For this review, take the finished solid that the model builds, in its own axes (mm). Face numbers are marked on the shaded views. A direction names the side the tool comes from. Round coordinates to 2 decimals unless told otherwise and drop trailing zeros. Write each loop counter-clockwise with the first axis right and the second up, starting at its lowest first coordinate (ties: lowest second). Pieces come first, ordered by that corner, then holes. Notation, with made-up numbers: (-28, 74.25) - (9, 74.25) arc R4 ccw to (9, 79.25) - close; hole circle Ø5 at (26, 79.5). An arc over 180 degrees is marked (long way). Answer in a Markdown table with one row per item. Add a question column.
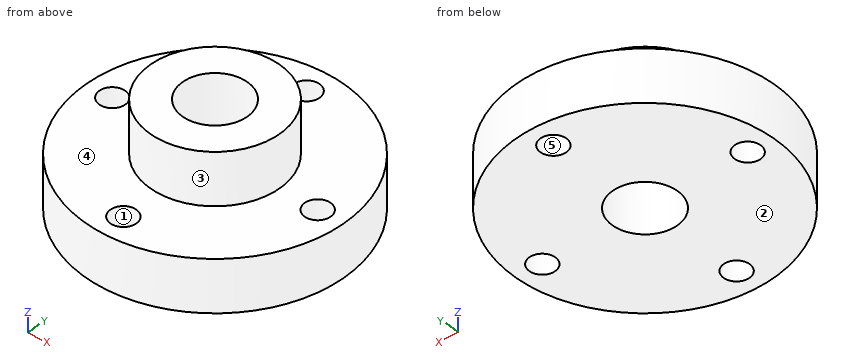
from build123d import *

# Parameters (mm, degrees)
F0_W     = 15.875
F0_H     = 12.7
F2_R     = 7.9375
F3_DEPTH = 25.401
F4_R     = 3.175
F5_DEPTH = 12.701


with BuildPart() as f1:
    # F0 (on Front) → F1 (revolve)
    with BuildSketch(Plane.XZ):
        Polygon((-31.75, 0), (0, 0), (0, 12.7), (-15.875, 12.7), (-31.75, 12.7), align=None)
        with Locations((-7.9375, 19.05)):
            Rectangle(F0_W, F0_H)
    revolve(axis=Axis((0, 0, 2.126115), (0, 0, -1)))

    # F2 (on face) → F3 (cut, through all)
    with BuildSketch(Plane.XY.offset(25.4)):
        Circle(F2_R)
    extrude(amount=-F3_DEPTH, mode=Mode.SUBTRACT)

    # F4 (on face) → F5 (cut, through all)
    with BuildSketch(Plane.XY.offset(12.7)):
        with Locations((0, 25.4)):
            Circle(F4_R)
        with Locations((25.4, 0)):
            Circle(F4_R)
        with Locations((0, -25.4)):
            Circle(F4_R)
        with Locations((-25.4, 0)):
            Circle(F4_R)
    extrude(amount=-F5_DEPTH, mode=Mode.SUBTRACT)


solid = f1.part
Q1. Draft analysis for pull direction Y (two halves, no side actions). For the marked faces 1, 2 and 3, state which applies: released by +Y, released by -Y, zero draft, split by the parting line, or undercut.
Q2. Add section C-C on z = 4.5. Count the separate pieces of the cut face and the enclosed holes in it, then the cut area to 3 significant figures.
Q3. To check wall thickness, follow probe 1 along Z at (x, y) = (27, 5.5); probe 2 along Y at (x, z) = (25.4, 2.5) (3 decimals); probe 3 along X at (y, z) = (-2, 6.5). State the ranges of each line that lie inside material, in increasing order.
Q4. Tool access review of the marked faces 4 and 5: name each direction out of +Z, -Z, +X, -X, +Y, -Y from which nothing blocks a thin tool from reaching the whole face with its end or side.
Q5. Insertion check: pin 1 Ø2 at (x, y) = (-18.5, -12.5) entering from +Z; pin 2 Ø1 at (y, z) = (24, 8.5) entering from +X; pin 3 Ø2 at (x, z) = (19.5, 6) entering from +Y. Each pin has a flat end and moves straight along its axis. Give the tip position at first contact, or say it passes through.
Q6. Add section A-A on x = -25.4. State the section outline as (y, z) points (3 decimals).
Answer sheet:
| question | item | result |
|---|---|---|
| 1 | face 1 | undercut |
| 1 | face 2 | zero draft |
| 1 | face 3 | split by the parting line |
| 2 | separate pieces | 1 |
| 2 | enclosed holes | 5 |
| 2 | area | 2,840 mm² |
| 3 | probe 1 | z = 0 to 12.7 |
| 3 | probe 2 | y = -19.05 to -3.175, 3.175 to 19.05 |
| 3 | probe 3 | x = -31.69 to -27.87, -22.93 to -7.68, 7.68 to 22.93, 27.87 to 31.69 |
| 4 | face 4 | +Z |
| 4 | face 5 | +Z, -Z |
| 5 | pin 1 | stops at z = 12.7 |
| 5 | pin 2 | stops at x = 21.35 |
| 5 | pin 3 | stops at y = 25.8 |
| 6 | outline | (-19.05, 0) - (-3.175, 0) - (-3.175, 12.7) - (-19.05, 12.7) - close; (3.175, 0) - (19.05, 0) - (19.05, 12.7) - (3.175, 12.7) - close |
